```python
from build123d import *

# Parameters (mm, degrees)
SKETCH1_R           = 3.96875
BOSS_EXTRUDE1_DEPTH = 153.9875
SKETCH2_R           = 1.55575
CUT_EXTRUDE1_DEPTH  = 309.02613944


with BuildPart() as part:
    # Sketch1 → Boss-Extrude1 (new, symmetric)
    with BuildSketch(Plane(origin=(0, 0, 0), x_dir=(0, 0, -1), z_dir=(1, 0, 0))):
        Circle(SKETCH1_R)
    extrude(amount=BOSS_EXTRUDE1_DEPTH, both=True)

    # Sketch6 → #10-32 Tapped Hole1 (revolve, cut)
    with BuildSketch(Plane(origin=(-153.9875, 0, 0), x_dir=(0, 0, 1), z_dir=(0, 1, 0))):
        Polygon((0, 0), (0, 26.613317848), (2.0193, 25.4), (2.0193, 0), align=None)
    f_10_32_tapped_hole1 = revolve(axis=Axis((-160.3375, 0, 0), (1, 0, 0)), mode=Mode.SUBTRACT)

    # Sketch2 → Cut-Extrude1 (cut, through all)
    with BuildSketch(Plane(origin=(153.9875, 0, 0), x_dir=(0, 0, -1), z_dir=(1, 0, 0))):
        Circle(SKETCH2_R)
    extrude(amount=-CUT_EXTRUDE1_DEPTH, mode=Mode.SUBTRACT)

    # Mirror1: #10-32 Tapped Hole1 across plane
    add(f_10_32_tapped_hole1.mirror(Plane(origin=(0, 0, 0), x_dir=(0, 0, 1), z_dir=(1, 0, 0))), mode=Mode.SUBTRACT)


solid = part.part
```
Could you check a few things on this model? Use its own coordinates, in mm. Round coordinates to 2 decimals unless told otherwise and drop trailing zeros. Write each loop counter-clockwise with the first axis right and the second up, starting at its lowest first coordinate (ties: lowest second). Pieces come first, ordered by that corner, then holes. Notation, with made-up numbers: M 30,-38 L 77,-38 A16 ccw 77,-16 Z; hole C 71.25,-17.5 d3. An arc over 180 degrees is marked long. Write each question's results on one line, items separated by ' | '. Start each with the question number.
1. Imagine slicing it at D-D on x = -31. List the corners of the cut face in (y, z) for me, and give its area (3 significant figures).
2. Imagine slicing it at C-C on x = -134. List the corners of the cut face in (y, z) for me, and give its area (3 significant figures).
3. I need wall thicknesses on L1, parallel to Y at x = -136, z = 0; L2, parallel to Z at x = 78.5, y = -0.25; L3, parallel to Z at x = 95, y = 1. Which ranges of each line are inside material? Lowest first, please. Write a range as from..to.
4. Imagine slicing it at A-A on z = 0. List the corners of the cut face in (x, y) for me.
5. I'm going to push flat-ended pins straight in: pin 1 Ø1.5 at (x, z) = (17.5, -1) entering from +Y; pin 2 Ø1.5 at (x, y) = (6, -2) entering from -Z. Where does each tip first touch, or does it pass through?
Result sheet:
1) outline: C 0,0 d7.94; hole C 0,0 d3.11 | area: 41.9 mm^2
2) outline: C 0,0 d7.94; hole C 0,0 d4.04 | area: 36.7 mm^2
3) L1: y = -3.97..-2.02, 2.02..3.97 | L2: z = -3.96..-1.54, 1.54..3.96 | L3: z = -3.84..-1.19, 1.19..3.84
4) outline: M -153.99,-3.97 L 153.99,-3.97 L 153.99,-2.02 L 128.59,-2.02 L 128.31,-1.56 L -128.31,-1.56 L -128.59,-2.02 L -153.99,-2.02 Z; M -153.99,2.02 L -128.59,2.02 L -128.31,1.56 L 128.31,1.56 L 128.59,2.02 L 153.99,2.02 L 153.99,3.97 L -153.99,3.97 Z
5) pin 1: stops at y = 3.96 | pin 2: stops at z = -3.77
